Check sheet for the modelled part. Datum: model origin and axes. Units: mm. Face numbers are marked on the shaded views. Coordinates: 2 decimals unless noted, no trailing zeros. Loops run counter-clockwise (first coordinate to the right, second up) from the corner with the lowest first, then second, coordinate; pieces in that order, holes last. Notation, with made-up numbers: (36, 62.5) - (68, 62.5) arc R20 ccw to (68, 66.5) - close; hole circle Ø2 at (-7.5, 51.5). An arc over 180 degrees is marked (long way). Use a Markdown table: item, result. Add a question column.
1) Sectioned sample at C-C, the plane y = 33.5. Enter the section's corners in (x, z), then the cut area to 3 significant figures.
2) Thickness scan on line 1 (Y direction, x = -22.5, z = 23.5); line 2 (X direction, y = 4, z = 15.25); line 3 (X direction, y = -18, z = 23.5). Record the ranges inside material, lowest first.
3) Sectioned sample at B-B, the plane x = -20. Enter the section's corners in (y, z), then the cut area to 3 significant figures.
4) Draft check along X on the marked faces 1, 2, 3 and 4. Enter one of: pulls with the +X half, pulls with the -X half, needs draft (parallel to the pull), parting line crosses it, or undercut.
5) Go/stop test with flat-tipped pins: P1, Ø1.3, axis at y = 66, z = 12.5, coming from the -X side; P2, Ø6, axis at x = -4, z = 14.5, coming from the +Y side; P3, Ø1.5, axis at x = -50, y = -21, coming from the +Z side. Record where each tip stops, or that it passes through.
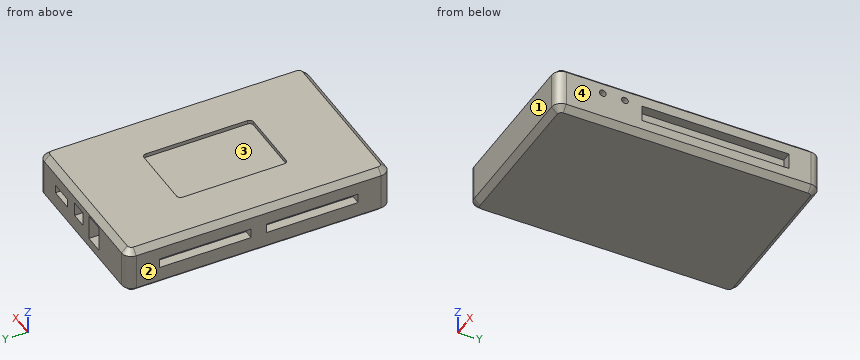
from build123d import *

# Parameters (mm, degrees)
F0_W      = 86
F0_H      = 136.6
F1_DEPTH  = 24.7
F3_R      = 5
F4_SIZE   = 3
F6_DEPTH  = 2
F7_W      = 47.5
F7_H      = 5
F8_DEPTH  = 5
F2_W      = 12
F2_H      = 4.5
F2_W_2    = 8.5
F2_H_2    = 7.3
F2_W_3    = 10
F2_H_3    = 13
F9_DEPTH  = 10
F10_W     = 76
F10_H     = 8.4
F10_R     = 1.75
F11_DEPTH = 5


with BuildPart() as f1:
    # F0 (on Top) → F1 (new body)
    with BuildSketch(Plane.XY):
        with Locations((-8.874781, 1.473147)):
            Rectangle(F0_W, F0_H)
    extrude(amount=F1_DEPTH)

    # F3
    f3_edges = [f1.edges().sort_by_distance(p)[0] for p in [
        (-51.874781, -66.826853, 12.35),
        (34.125219, -66.826853, 12.35),
        (34.125219, 69.773147, 12.35),
        (-51.874781, 69.773147, 12.35),
    ]]
    fillet(f3_edges, radius=F3_R)

    # F4
    f4_edges = [f1.edges().sort_by_distance(p)[0] for p in [
        (34.125219, 1.473147, 24.7),
        (32.660753, -65.362386, 24.7),
        (32.660753, 68.308681, 24.7),
        (-8.874781, -66.826853, 24.7),
        (-8.874781, 69.773147, 24.7),
        (-50.410315, -65.362386, 24.7),
        (-50.410315, 68.308681, 24.7),
        (-51.874781, 1.473147, 24.7),
        (34.125219, 1.473147, 0),
        (32.660753, -65.362386, 0),
        (32.660753, 68.308681, 0),
        (-8.874781, -66.826853, 0),
        (-8.874781, 69.773147, 0),
        (-50.410315, -65.362386, 0),
        (-50.410315, 68.308681, 0),
        (-51.874781, 1.473147, 0),
    ]]
    chamfer(f4_edges, length=F4_SIZE)

    # F5 (on face) → F6 (cut)
    with BuildSketch(Plane.XY.offset(24.7)):
        with BuildLine():
            Line((7.125219, 29.773147), (-24.874781, 29.773147))
            ThreePointArc((-24.874781, 29.773147), (-26.288994, 29.187361), (-26.874781, 27.773147))
            Line((-26.874781, 27.773147), (-26.874781, -24.826853))
            ThreePointArc((-26.874781, -24.826853), (-26.288994, -26.241066), (-24.874781, -26.826853))
            Line((-24.874781, -26.826853), (7.125219, -26.826853))
            ThreePointArc((7.125219, -26.826853), (8.539433, -26.241066), (9.125219, -24.826853))
            Line((9.125219, -24.826853), (9.125219, 27.773147))
            ThreePointArc((9.125219, 27.773147), (8.539433, 29.187361), (7.125219, 29.773147))
        make_face()
    extrude(amount=-F6_DEPTH, mode=Mode.SUBTRACT)

    # F7 (on face) → F8 (cut)
    with BuildSketch(Plane(origin=(-51.874781, 0, 0), x_dir=(0, -1, 0), z_dir=(-1, 0, 0))):
        with Locations((-29.123147, 12.9)):
            Rectangle(F7_W, F7_H)
        with Locations((26.176853, 12.9)):
            Rectangle(F7_W, F7_H)
    extrude(amount=-F8_DEPTH, mode=Mode.SUBTRACT)

    # F2 (on face) → F9 (cut)
    with BuildSketch(Plane(origin=(0, 69.773147, 0), x_dir=(-1, 0, 0), z_dir=(0, 1, 0))):
        with Locations((-12.125219, 13.4)):
            Rectangle(F2_W, F2_H)
        with Locations((4.874781, 14.8)):
            Rectangle(F2_W_2, F2_H_2)
        with Locations((19.774781, 14.15)):
            Rectangle(F2_W_3, F2_H_3)
    extrude(amount=-F9_DEPTH, mode=Mode.SUBTRACT)

    # F10 (on face) → F11 (cut)
    with BuildSketch(Plane.YZ.offset(34.125219)):
        with Locations((15.273147, 12.2)):
            Rectangle(F10_W, F10_H)
        with Locations((-42.926853, 16.4)):
            Circle(F10_R)
        with Locations((-31.526853, 16.4)):
            Circle(F10_R)
    extrude(amount=-F11_DEPTH, mode=Mode.SUBTRACT)


solid = f1.part
Solved:
| question | item | result |
|---|---|---|
| 1 | outline | (-51.87, 3) - (-48.87, 0) - (31.13, 0) - (34.13, 3) - (34.13, 8) - (29.13, 8) - (29.13, 16.4) - (34.13, 16.4) - (34.13, 21.7) - (31.13, 24.7) - (-48.87, 24.7) - (-51.87, 21.7) - (-51.87, 15.4) - (-46.87, 15.4) - (-46.87, 10.4) - (-51.87, 10.4) - close |
| 1 | area | 2,040 mm2 |
| 2 | line 1 | y = -65.03 to -26.83, 29.77 to 67.97 |
| 2 | line 2 | x = -51.87 to 29.13 |
| 2 | line 3 | x = -50.07 to -26.87, 9.13 to 32.33 |
| 3 | outline | (-66.83, 3) - (-63.83, 0) - (66.77, 0) - (69.77, 3) - (69.77, 7.65) - (59.77, 7.65) - (59.77, 20.65) - (69.77, 20.65) - (69.77, 21.7) - (66.77, 24.7) - (29.77, 24.7) - (29.77, 22.7) - (-26.83, 22.7) - (-26.83, 24.7) - (-63.83, 24.7) - (-66.83, 21.7) - close |
| 3 | area | 3,110 mm2 |
| 4 | face 1 | needs draft |
| 4 | face 2 | pulls with the -X half |
| 4 | face 3 | undercut |
| 4 | face 4 | pulls with the +X half |
| 5 | P1 | stops at x = -51.84 |
| 5 | P2 | stops at y = 59.77 |
| 5 | P3 | stops at z = 24.32 |
